Check sheet for the modelled part. Datum: model origin and axes. Units: mm. Face numbers are marked on the shaded views. A direction names the side the tool comes from. Give positions to 0.01 mm unless a question says otherwise; leave off trailing zeros. Order: outer loops, then holes, each group sorted by start corner. A loop starts at its lowest first (then second) coordinate and runs counter-clockwise, first axis right, second up.
Item 1: Sectioned sample at A-A on z = 25. Record the boundary of the cut face in (x, y), and give its area (3 significant figures).
Item 2: Sectioned sample at B-B on y = 10. Record the boundary of the cut face in (x, z), and give its area (3 significant figures).
Item 3: Sectioned sample at C-C on x = 365.5. Record the boundary of the cut face in (y, z), and give its area (3 significant figures).
Item 4: Material ranges on line 1 along Z through (x, y) = (242, 9); line 2 along Z through (x, y) = (164.5, 4.5), recorded low to high.
Item 5: Access from +Z, -Z, +X, -X, +Y, -Y to the whole of each face (thin tool, end or side, straight path). Record for the marked faces 1 and 2.
Item 6: Sectioned sample at D-D on z = 4. Record the boundary of the cut face in (x, y), and give its area (3 significant figures).
Item 7: Gauge pin test, flat ends, axial feed: P1, Ø5, axis at x = 378.5, z = -1.5, coming from the +Y side; P2, Ø7.5, axis at x = 175, y = 10, coming from the +Z side; P3, Ø4, axis at y = 2, z = 22, coming from the +X side. Record the tip position at first contact, or that the pin passes through.
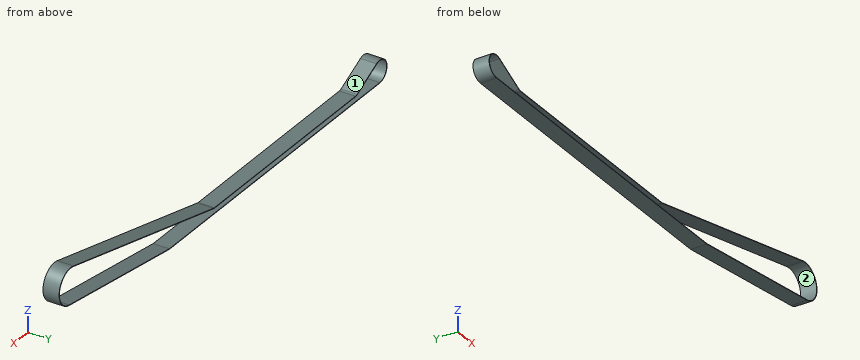
from build123d import *

# Parameters (mm, degrees)
BOSS_EXTRUDE1_DEPTH = 15


with BuildPart() as part:
    # Sketch2 → Boss-Extrude1 (new body)
    with BuildSketch(Plane(origin=(0, 0, 0), x_dir=(1, 0, 0), z_dir=(0, 1, 0))):
        with BuildLine():
            Line((0, 10.5), (303.9759017, 10.5))
            Line((303.9759017, 10.5), (448.913075843, -10.421830981))
            ThreePointArc((448.913075843, -10.421830981), (462.973791064, -30.136121747), (442.647176825, -43.296126554))
            Line((442.647176825, -43.296126554), (239.996066619, 4.864515389))
            ThreePointArc((239.996066619, 4.864515389), (239.421989284, 4.966013338), (238.84, 5))
            Line((238.84, 5), (35, 5))
            ThreePointArc((35, 5), (33.863075353, 4.869024784), (32.785714286, 4.482960938))
            Line((32.785714286, 4.482960938), (4.65, -9.414217971))
            ThreePointArc((4.65, -9.414217971), (-10.224952046, -2.38754176), (0, 10.5))
        make_face()
        with BuildLine():
            Line((0, 10), (303.94, 10))
            Line((303.94, 10), (448.841640743, -10.916701698))
            ThreePointArc((448.841640743, -10.916701698), (462.482633122, -30.042506173), (442.762783487, -42.809675015))
            Line((442.762783487, -42.809675015), (240.111673281, 5.350966928))
            ThreePointArc((240.111673281, 5.350966928), (239.480188213, 5.462614672), (238.84, 5.5))
            Line((238.84, 5.5), (35, 5.5))
            ThreePointArc((35, 5.5), (33.749382888, 5.355927262), (32.564285714, 4.931257032))
            Line((32.564285714, 4.931257032), (4.428571429, -8.965921877))
            ThreePointArc((4.428571429, -8.965921877), (-9.738049568, -2.273849295), (0, 10))
        make_face(mode=Mode.SUBTRACT)
    extrude(amount=BOSS_EXTRUDE1_DEPTH)


solid = part.part
Report:
1. outline: (365.66, 0) - (367.82, 0) - (367.82, 15) - (365.66, 15) - close; (462.65, 0) - (463.15, 0) - (463.15, 15) - (462.65, 15) - close
1. area: 40.0 mm2
2. outline: (0, -10.5) - (303.98, -10.5) - (448.91, 10.42) arc R16.75 ccw (long way) to (442.65, 43.3) - (240, -4.86) arc R5 cw to (238.84, -5) - (35, -5) arc R5 cw to (32.79, -4.48) - (4.65, 9.41) arc R10.5 ccw (long way) to start; hole (0, -10) - (303.94, -10) - (448.84, 10.92) arc R16.25 ccw (long way) to (442.76, 42.81) - (240.11, -5.35) arc R5.5 cw to (238.84, -5.5) - (35, -5.5) arc R5.5 cw to (32.56, -4.93) - (4.43, 8.97) arc R10 ccw (long way) to start
2. area: 494 mm2
3. outline: (0, -1.62) - (15, -1.62) - (15, -1.11) - (0, -1.11) - close; (0, 24.45) - (15, 24.45) - (15, 24.96) - (0, 24.96) - close
3. area: 15.3 mm2
4. line 1: z = -10.5 to -10, -4.9 to -4.39
4. line 2: z = -10.5 to -10, -5.5 to -5
5. face 1: +Z, +Y, -Y
5. face 2: +Y, -Y
6. outline: (-9.71, 0) - (-9.17, 0) - (-9.17, 15) - (-9.71, 15) - close; (14.48, 0) - (15.61, 0) - (15.61, 15) - (14.48, 15) - close; (277.3, 0) - (279.46, 0) - (279.46, 15) - (277.3, 15) - close; (400.93, 0) - (404.43, 0) - (404.43, 15) - (400.93, 15) - close
6. area: 110 mm2
7. P1: stops at y = 15
7. P2: stops at z = -5
7. P3: stops at x = 463
